Source: three-view drawing plus pictorial views. Frame: mm from the lowest corner of the part. Give positions to 0.01 mm unless a question says otherwise; leave off trailing zeros. Loops run counter-clockwise (first coordinate to the right, second up) from the corner with the lowest first, then second, coordinate; pieces in that order, holes last. Notation, with made-up numbers: (41, 44) -> (78, 44) arc R32 ccw to (78, 74) -> close; hole circle Ø10 at (58, 75). An arc over 180 degrees is marked (long way). One line per item, written item: value. Start each with the question number.
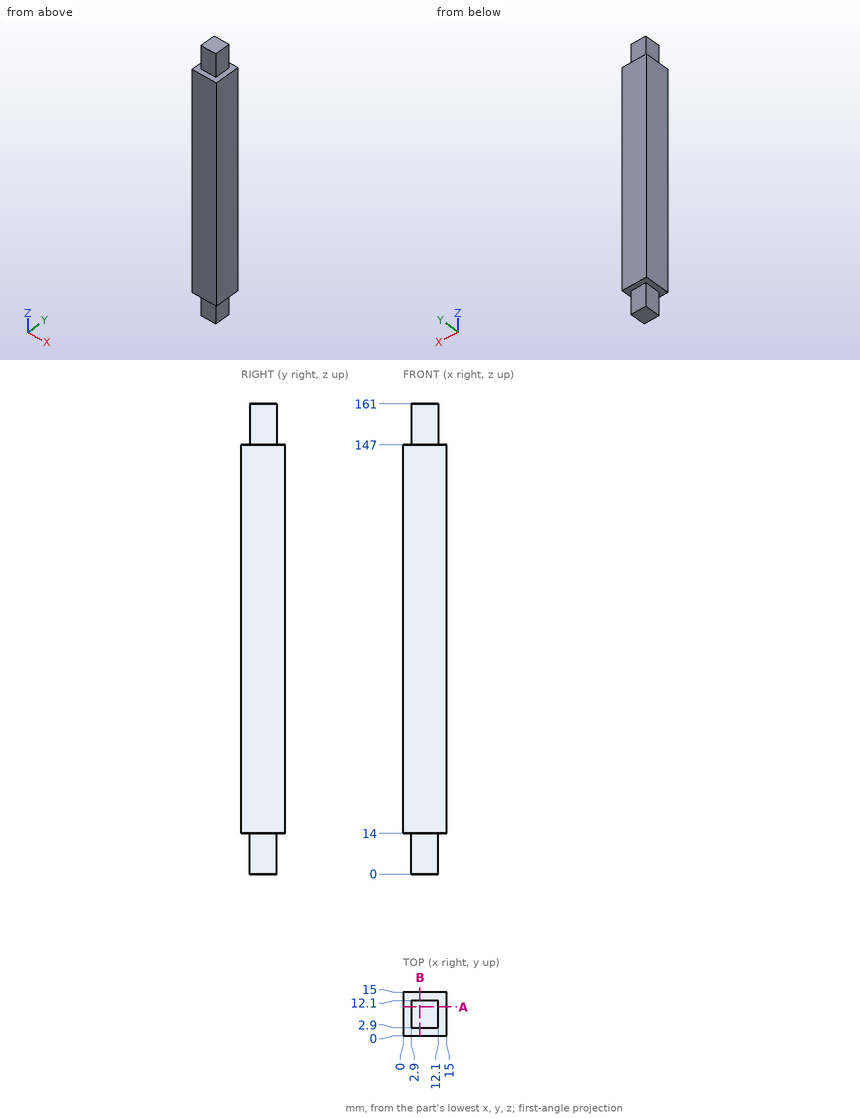
Item 1: Section A-A, the plane y = 10. Output: boundary loops of the cut face in (x, z).
Item 2: Pin query (flat end, axial travel): pin 1 (7.5 mm diameter, centred on x = 7, z = 155.5, fed in from +Y); pin 2 (4.5 mm diameter, centred on y = 9.5, z = 10, fed in from -X); pin 3 (3 mm diameter, centred on y = 6.5, z = 157, fed in from +X). Return the tip coordinate at first contact, or that it passes through.
Item 3: Ray query, line 1 along Z through (x, y) = (13, 4.75); line 2 along Y through (x, z) = (11.5, 149.5). Return the intervals inside material, ascending. Write a range as [from, to].
Geometry check:
1. outline: (0, 14) -> (2.9, 14) -> (2.9, 0) -> (12.1, 0) -> (12.1, 14) -> (15, 14) -> (15, 147) -> (12.1, 147) -> (12.1, 161) -> (2.9, 161) -> (2.9, 147) -> (0, 147) -> close
2. pin 1: stops at y = 12.1
2. pin 2: stops at x = 2.9
2. pin 3: stops at x = 12.1
3. line 1: z = [14, 147]
3. line 2: y = [2.9, 12.1]
